Design review of the part built by this model. Coordinates are the model's own, in mm. Face numbers are marked on the shaded views. A direction names the side the tool comes from. Coordinates: 2 decimals unless noted, no trailing zeros. Write each loop counter-clockwise with the first axis right and the second up, starting at its lowest first coordinate (ties: lowest second). Pieces come first, ordered by that corner, then holes. Notation, with made-up numbers: (-32, 44.25) - (11, 44.25) arc R5 ccw to (11, 50.25) - close; hole circle Ø9 at (19.5, -36.5). An arc over 180 degrees is marked (long way). Use a Markdown table: item, result.
from build123d import *

# Parameters (mm, degrees)
SKETCH_1_W          = 16.22
SKETCH_1_H          = 8.42
EXTRUDE_1_DEPTH     = 11
SKETCH_2_R          = 0.86
EXTRUDE_2_DEPTH     = 0.68
SKETCH_3_W          = 16.22
SKETCH_3_H          = 8.42
EXTRUDE_3_DEPTH     = 3.44
EXTRUDE_4_DEPTH     = 2.61
EXTRUDE_5_DEPTH     = 0.58
SKETCH_6_R          = 1.89
EXTRUDE_6_DEPTH     = 5.38
SKETCH_7_R          = 0.585
CUT_EXTRUDE_1_DEPTH = 3.6
FILLET_START        = -17
FILLET_1_OUTLINE_W  = 5
FILLET_1_OUTLINE_H  = 12
FILLET_1_DEPTH      = 1.938625561
FILLET_1_2_R        = 0.3
SKETCH_8_W          = 3.84
SKETCH_8_H          = 2.845310476
EXTRUDE_7_DEPTH     = 0.62


with BuildPart() as part:
    # Sketch 1 → Extrude 1 (new body)
    with BuildSketch(Plane(origin=(0, 0, 0), x_dir=(1, 0, 0), z_dir=(0, 1, 0))):
        Rectangle(SKETCH_1_W, SKETCH_1_H)
    extrude(amount=EXTRUDE_1_DEPTH)

    # Sketch 2 → Extrude 2 (add)
    # profile 1 of 2: a face of its own
    with BuildSketch(Plane(origin=(0, 11, 0), x_dir=(1, 0, 0), z_dir=(0, 1, 0))):
        with BuildLine():
            Line((-8.11, -4.21), (-8.11, 4.21))
            Line((-8.11, 4.21), (-9.82, 4.21))
            ThreePointArc((-9.82, 4.21), (-11.55, 0), (-9.82, -4.21))
            Line((-9.82, -4.21), (-8.11, -4.21))
        make_face()
        with Locations(Location((-9.82, 0, 0), (0, 0, 270))):
            Circle(SKETCH_2_R, mode=Mode.SUBTRACT)
    # profile 2 of 2: a face of its own
    with BuildSketch(Plane(origin=(0, 11, 0), x_dir=(1, 0, 0), z_dir=(0, 1, 0))):
        with BuildLine():
            Line((9.82, 4.21), (8.11, 4.21))
            Line((8.11, 4.21), (8.11, -4.21))
            Line((8.11, -4.21), (9.82, -4.21))
            ThreePointArc((9.82, -4.21), (11.55, 0), (9.82, 4.21))
        make_face()
        with Locations(Location((9.82, 0, 0), (0, 0, 270))):
            Circle(SKETCH_2_R, mode=Mode.SUBTRACT)
    extrude(amount=-EXTRUDE_2_DEPTH)

    # Sketch 3 → Extrude 3 (add)
    with BuildSketch(Plane(origin=(0, 11, 0), x_dir=(1, 0, 0), z_dir=(0, 1, 0))):
        Rectangle(SKETCH_3_W, SKETCH_3_H)
    extrude(amount=EXTRUDE_3_DEPTH)

    # Sketch 4 → Extrude 4 (add)
    with BuildSketch(Plane(origin=(0, 14.44, 0), x_dir=(1, 0, 0), z_dir=(0, 1, 0))):
        with BuildLine():
            ThreePointArc((0.516921129, -2.35), (-0.2, 0), (0.516921129, 2.35))
            Line((0.516921129, 2.35), (-0.12, 2.35))
            ThreePointArc((-0.12, 2.35), (-2.47, 0), (-0.12, -2.35))
            Line((-0.12, -2.35), (0.516921129, -2.35))
        make_face()
        with BuildLine():
            Line((4.01, 1.9), (4.01, 2.35))
            Line((4.01, 2.35), (0.516921129, 2.35))
            ThreePointArc((0.516921129, 2.35), (-0.2, 0), (0.516921129, -2.35))
            Line((0.516921129, -2.35), (4.01, -2.35))
            Line((4.01, -2.35), (4.01, -1.9))
            ThreePointArc((4.01, -1.9), (2.11, 0), (4.01, 1.9))
        make_face()
        with BuildLine():
            Line((4.01, 2.35), (4.01, 4.21))
            ThreePointArc((4.01, 4.21), (2.031288298, 3.716019376), (0.516921129, 2.35))
            Line((0.516921129, 2.35), (4.01, 2.35))
        make_face()
        with BuildLine():
            ThreePointArc((0.516921129, -2.35), (2.031288298, -3.716019376), (4.01, -4.21))
            Line((4.01, -4.21), (4.01, -2.35))
            Line((4.01, -2.35), (0.516921129, -2.35))
        make_face()
        with BuildLine():
            Line((8.11, -4.21), (8.11, 4.21))
            Line((8.11, 4.21), (4.01, 4.21))
            Line((4.01, 4.21), (4.01, 2.35))
            Line((4.01, 2.35), (4.18798505, 2.35))
            ThreePointArc((4.18798505, 2.35), (6.53798505, 0), (4.18798505, -2.35))
            Line((4.18798505, -2.35), (4.01, -2.35))
            Line((4.01, -2.35), (4.01, -4.21))
            Line((4.01, -4.21), (8.11, -4.21))
        make_face()
        with BuildLine():
            Line((4.18798505, 2.35), (4.01, 2.35))
            Line((4.01, 2.35), (4.01, 1.9))
            ThreePointArc((4.01, 1.9), (5.353502884, 1.343502884), (5.91, 0))
            ThreePointArc((5.91, 0), (5.353502884, -1.343502884), (4.01, -1.9))
            Line((4.01, -1.9), (4.01, -2.35))
            Line((4.01, -2.35), (4.18798505, -2.35))
            ThreePointArc((4.18798505, -2.35), (6.53798505, 0), (4.18798505, 2.35))
        make_face()
    extrude(amount=EXTRUDE_4_DEPTH)

    # Sketch 5 → Extrude 5 (add)
    with BuildSketch(Plane(origin=(0, 17.05, 0), x_dir=(1, 0, 0), z_dir=(0, 1, 0))):
        with BuildLine():
            Line((-1.11, 0.96), (-0.13, 0.96))
            ThreePointArc((-0.13, 0.96), (0.83, 0), (-0.13, -0.96))
            Line((-0.13, -0.96), (-1.11, -0.96))
            ThreePointArc((-1.11, -0.96), (-2.07, 0), (-1.11, 0.96))
        make_face()
    extrude(amount=EXTRUDE_5_DEPTH)

    # Sketch 6 → Extrude 6 (add)
    with BuildSketch(Plane(origin=(0, 14.44, 0), x_dir=(1, 0, 0), z_dir=(0, 1, 0))):
        with Locations(Location((4.01, 0, 0), (0, 0, 270))):
            Circle(SKETCH_6_R)
    extrude(amount=EXTRUDE_6_DEPTH)

    # Sketch 7 → Cut-Extrude 1 (cut)
    with BuildSketch(Plane(origin=(0, 19.82, 0), x_dir=(1, 0, 0), z_dir=(0, 1, 0))):
        with Locations(Location((4.01, 0, 0), (0, 0, 270))):
            Circle(SKETCH_7_R)
    extrude(amount=-CUT_EXTRUDE_1_DEPTH, mode=Mode.SUBTRACT)

    # Fillet 1: read off the stored shape, not the designer's step
    # Fillet 1 outline → Fillet 1 (cut)
    with BuildSketch(Plane(origin=(0, 0, 0), x_dir=(0.707106781186548, 0.707106781186547, 0), z_dir=(0.707106781186547, -0.707106781186548, 0)).offset(FILLET_START)):
        with Locations((4.5, 0)):
            Rectangle(FILLET_1_OUTLINE_W, FILLET_1_OUTLINE_H)
    extrude(amount=FILLET_1_DEPTH, mode=Mode.SUBTRACT)

    # Fillet 1 2
    fillet_1_2_edges = [part.edges().sort_by_distance(p)[0] for p in [
        (-8.11, 12.095, 4.21),
        (-8.11, 12.095, -4.21),
        (-8.11, 5.16, 4.21),
        (-8.11, 5.16, -4.21),
        (8.11, 5.16, -4.21),
        (8.11, 5.16, 4.21),
        (8.11, 14.025, -4.21),
        (8.11, 14.025, 4.21),
    ]]
    fillet(fillet_1_2_edges, radius=FILLET_1_2_R)

    # Sketch 8 → Extrude 7 (add)
    with BuildSketch(Plane(origin=(8.11, 0, 0), x_dir=(0, 0, -1), z_dir=(1, 0, 0))):
        with Locations((0, 2.857344762)):
            Rectangle(SKETCH_8_W, SKETCH_8_H)
    extrude(amount=EXTRUDE_7_DEPTH)


solid = part.part
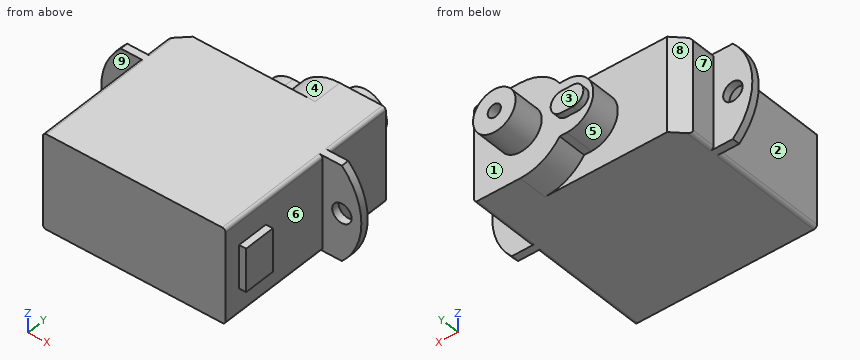
(1) For pin 1 (3 mm diameter, centred on x = -2.5, z = -2.5, fed in from +Y); pin 2 (4 mm diameter, centred on x = -2, z = 0.5, fed in from +Y); pin 3 (0.5 mm diameter, centred on x = -0.5, y = 17.5, fed in from -Z), all flat-tipped, find the tip position at first contact; note any pin that passes through.
Determined:
| item | result |
|---|---|
| pin 1 | y = 17.05 |
| pin 2 | y = 17.63 |
| pin 3 | z = -0.96 |
(2) Draft analysis for pull direction Y (two halves, no side actions). For the marked faces 6, 7, 8 and 9, state which applies: +Y half, -Y half, draft (parallel to the pull), parting line (faces both ways), or undercut.
Determined:
| item | result |
|---|---|
| face 6 | undercut |
| face 7 | draft |
| face 8 | +Y half |
| face 9 | -Y half |
(3) For L1, parallel to X at y = 1.5, z = 1.75; L2, parallel to Y at x = -2.5, z = -1.5; L3, parallel to X at y = 10.25, z = 3, list the stretches that pass through material, from the lowest coordinate up. Write a range as from..to.
Determined:
| item | result |
|---|---|
| L1 | -8.11..8.73 |
| L2 | 0..14.44 |
| L3 | -8.11..8.11 |
(4) Take a section at B-B on z = -3.5. Write out the cut boundary in (x, y).
Determined:
| item | result |
|---|---|
| outline | (-10.42, 10.32) - (-8.11, 10.32) - (-8.11, 0) - (8.11, 0) - (8.11, 10.32) - (10.42, 10.32) - (10.42, 11) - (8.11, 11) - (8.11, 17.05) - (1.67, 17.05) - (1.67, 14.44) - (-6.86, 14.44) - (-8.11, 13.19) - (-8.11, 11) - (-10.42, 11) - close |
(5) Take a section at A-A on y = 15. Write out the cut boundary in (x, z).
Determined:
| item | result |
|---|---|
| outline | (-0.12, -2.35) - (0.52, -2.35) arc R4.21 ccw to (4.01, -4.21) - (7.81, -4.21) arc R0.3 ccw to (8.11, -3.91) - (8.11, 3.91) arc R0.3 ccw to (7.81, 4.21) - (4.01, 4.21) arc R4.21 ccw to (0.52, 2.35) - (-0.12, 2.35) arc R2.35 ccw to start; circle Ø3.78 at (4.01, 0); hole circle Ø3.8 at (4.01, 0) |
(6) Machinability: for the marked faces 1, 2, 3, 4 and 5, which of the approach directions +Z, -Z, +X, -X, +Y, -Y give a long, thin tool a straight path to every point of the face, cutting with its end or side? Answer none if there is none.
Determined:
| item | result |
|---|---|
| face 1 | +Y |
| face 2 | +Z, -Z, -X, -Y |
| face 3 | +Z, -Z, -X, +Y |
| face 4 | +Z, -X, +Y |
| face 5 | -X, +Y |
